Design review of the part built by this model. Coordinates are the model's own, in mm. Face numbers are marked on the shaded views. A direction names the side the tool comes from. Round coordinates to 2 decimals unless told otherwise and drop trailing zeros. Loops run counter-clockwise (first coordinate to the right, second up) from the corner with the lowest first, then second, coordinate; pieces in that order, holes last. Notation, with made-up numbers: M -4.75,-29.5 L 21.25,-29.5 A27 ccw 21.25,-13.5 Z; hole C -18.5,27 d5. An arc over 180 degrees is marked long. Use a Markdown table: item, result.
from build123d import *

# Parameters (mm, degrees)
ESQUISSE1_W             = 20
ESQUISSE1_H             = 20
BOSS_EXTRU_1_DEPTH      = 4
ESQUISSE4_W             = 20
ESQUISSE4_H             = 20
ESQUISSE4_W_2           = 12
ESQUISSE4_H_2           = 12
BOSS_EXTRU_2_DEPTH      = 16
ESQUISSE6_R             = 5
ENL_V_MAT_EXTRU_3_DEPTH = 25
ESQUISSE5_R             = 5
ENL_V_MAT_EXTRU_4_DEPTH = 25
CHANFREIN1_SIZE         = 2


with BuildPart() as part:
    # Esquisse1 → Boss.-Extru.1 (new body)
    with BuildSketch(Plane(origin=(0, 0, 0), x_dir=(1, 0, 0), z_dir=(0, 1, 0))):
        Rectangle(ESQUISSE1_W, ESQUISSE1_H)
    extrude(amount=BOSS_EXTRU_1_DEPTH)

    # Esquisse4 → Boss.-Extru.2 (add)
    with BuildSketch(Plane(origin=(0, 4, 0), x_dir=(1, 0, 0), z_dir=(0, 1, 0))):
        Rectangle(ESQUISSE4_W, ESQUISSE4_H)
        Rectangle(ESQUISSE4_W_2, ESQUISSE4_H_2, mode=Mode.SUBTRACT)
    extrude(amount=BOSS_EXTRU_2_DEPTH)

    # Esquisse6 → Enlèv. mat.-Extru.3 (cut)
    with BuildSketch(Plane(origin=(10, 0, 0), x_dir=(0, 0, -1), z_dir=(1, 0, 0))):
        with Locations((0, 10)):
            Circle(ESQUISSE6_R)
    extrude(amount=-ENL_V_MAT_EXTRU_3_DEPTH, mode=Mode.SUBTRACT)

    # Esquisse5 → Enlèv. mat.-Extru.4 (cut)
    with BuildSketch(Plane.XY.offset(10)):
        with Locations((0, 10)):
            Circle(ESQUISSE5_R)
    extrude(amount=-ENL_V_MAT_EXTRU_4_DEPTH, mode=Mode.SUBTRACT)

    # Chanfrein1
    chanfrein1_edges = [part.edges().sort_by_distance(p)[0] for p in [
        (10, 10, -10),
        (10, 10, 10),
        (-10, 10, 10),
        (-10, 10, -10),
    ]]
    chamfer(chanfrein1_edges, length=CHANFREIN1_SIZE)


solid = part.part
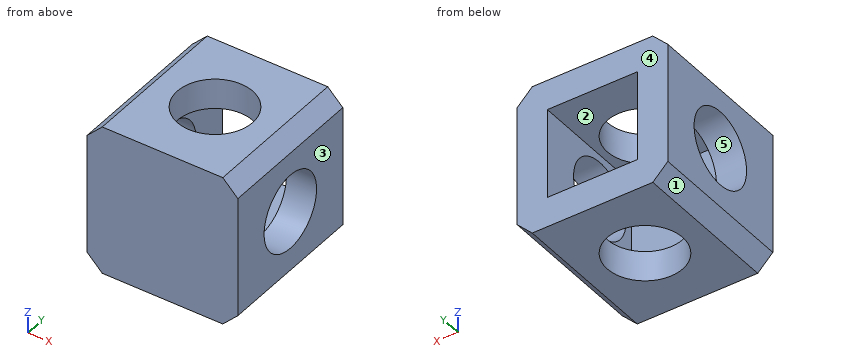
1. The part is to be moulded in two halves that separate along Y. For the marked faces 3, 4 and 5, say which applies: pulls with the +Y half, pulls with the -Y half, needs draft (parallel to the pull), parting line crosses it, or undercut.
Check values:
| item | result |
|---|---|
| face 3 | needs draft |
| face 4 | pulls with the +Y half |
| face 5 | undercut |
2. Machinability: for the marked faces 1 and 2, which of the approach directions +Z, -Z, +X, -X, +Y, -Y give a long, thin tool a straight path to every point of the face, cutting with its end or side? Answer none if there is none.
Check values:
| item | result |
|---|---|
| face 1 | -Z, -X, +Y, -Y |
| face 2 | +Y |
3. Take a section at C-C on x = 0. Give the boundary of the cut face in (y, z), and give its area (3 significant figures).
Check values:
| item | result |
|---|---|
| outline | M 0,-10 L 5,-10 L 5,-6 L 4,-6 L 4,6 L 5,6 L 5,10 L 0,10 Z; M 15,-10 L 20,-10 L 20,-6 L 15,-6 Z; M 15,6 L 20,6 L 20,10 L 15,10 Z |
| area | 128 mm² |
4. Insertion check: pin 1 (6 mm diameter, centred on x = 0, y = 10, fed in from -Z); pin 2 (4 mm diameter, centred on x = -1.5, z = -3.5, fed in from +Y). Each pin has a flat end and moves straight along its axis. Give the tip position at first contact, or say it passes through.
Check values:
| item | result |
|---|---|
| pin 1 | passes through |
| pin 2 | stops at y = 4 |
5. Wall thickness on line 1 along X through (y, z) = (16.75, 2.5); line 2 along Y through (x, z) = (0, 8.2): over which ranges is each line inside the solid? List them lowest first. Write a range as from..to.
Check values:
| item | result |
|---|---|
| line 1 | x = -10..-6, 6..10 |
| line 2 | y = 0..5, 15..20 |
6. Take a section at B-B on z = 0. Give the boundary of the cut face in (x, y).
Check values:
| item | result |
|---|---|
| outline | M -10,0 L 10,0 L 10,5 L 6,5 L 6,4 L -6,4 L -6,5 L -10,5 Z; M -10,15 L -6,15 L -6,20 L -10,20 Z; M 6,15 L 10,15 L 10,20 L 6,20 Z |
7. Take a section at A-A on y = 6. Give the boundary of the cut face in (x, z).
Check values:
| item | result |
|---|---|
| outline | M -10,-8 L -8,-10 L -3,-10 L -3,-6 L -6,-6 L -6,-3 L -10,-3 Z; M -10,3 L -6,3 L -6,6 L -3,6 L -3,10 L -8,10 L -10,8 Z; M 3,-10 L 8,-10 L 10,-8 L 10,-3 L 6,-3 L 6,-6 L 3,-6 Z; M 3,6 L 6,6 L 6,3 L 10,3 L 10,8 L 8,10 L 3,10 Z |
8. Take a section at D-D on y = 17. Give the boundary of the cut face in (x, z), and give its area (3 significant figures).
Check values:
| item | result |
|---|---|
| outline | M -10,-8 L -8,-10 L 8,-10 L 10,-8 L 10,8 L 8,10 L -8,10 L -10,8 Z; hole M -6,-6 L 6,-6 L 6,6 L -6,6 Z |
| area | 248 mm² |
